The model under review builds one solid part; all positions refer to its coordinate system, in mm. Round coordinates to 2 decimals unless told otherwise and drop trailing zeros. Write each loop counter-clockwise with the first axis right and the second up, starting at its lowest first coordinate (ties: lowest second). Pieces come first, ordered by that corner, then holes. Notation, with made-up numbers: (23, 22) - (73, 22) arc R17 ccw to (73, 31) - close; hole circle Ø4 at (19, -6.5). An arc over 180 degrees is marked (long way). Use one line per item in the form item = value.
from build123d import *

# Parameters (mm, degrees)
SKETCH_1_W          = 31.5
SKETCH_1_H          = 31.5
EXTRUDE_1_DEPTH     = 0.2
SKETCH_2_R          = 4.5
CUT_EXTRUDE_1_DEPTH = 10
SKETCH_3_R          = 1.5
SKETCH_3_R_2        = 4.5
CUT_EXTRUDE_2_DEPTH = 0.2


with BuildPart() as part:
    # 스케치1 → 보스-돌출1 (new body)
    with BuildSketch(Plane.XY):
        with Locations((15.75, 15.75)):
            Rectangle(SKETCH_1_W, SKETCH_1_H)
    extrude(amount=EXTRUDE_1_DEPTH)

    # 스케치2 → 컷-돌출1 (cut)
    with BuildSketch(Plane.XY.offset(0.2)):
        with Locations((15.75, 15.75)):
            Circle(SKETCH_2_R)
    extrude(amount=-CUT_EXTRUDE_1_DEPTH, mode=Mode.SUBTRACT)

    # 스케치3 → 컷-돌출2 (cut)
    with BuildSketch(Plane.XY.offset(0.2)):
        with Locations((29.7, 15.75)):
            Circle(SKETCH_3_R)
        with Locations((15.75, 15.75)):
            Circle(SKETCH_3_R_2)
        with Locations((15.75, 1.8)):
            Circle(SKETCH_3_R)
        with Locations((1.8, 15.75)):
            Circle(SKETCH_3_R)
        with Locations((15.75, 29.7)):
            Circle(SKETCH_3_R)
        with Locations((1.8, 29.7)):
            Circle(SKETCH_3_R)
        with Locations((29.7, 29.7)):
            Circle(SKETCH_3_R)
        with Locations((29.7, 1.8)):
            Circle(SKETCH_3_R)
        with Locations((1.8, 1.8)):
            Circle(SKETCH_3_R)
    extrude(amount=-CUT_EXTRUDE_2_DEPTH, mode=Mode.SUBTRACT)


solid = part.part
(1) Add section C-C on y = 1.8. Write out the cut boundary in (x, z).
Geometry results:
outline = (0, 0) - (0.3, 0) - (0.3, 0.2) - (0, 0.2) - close; (3.3, 0) - (14.25, 0) - (14.25, 0.2) - (3.3, 0.2) - close; (17.25, 0) - (28.2, 0) - (28.2, 0.2) - (17.25, 0.2) - close; (31.2, 0) - (31.5, 0) - (31.5, 0.2) - (31.2, 0.2) - close
(2) Add section B-B on x = 15.75. Write out the cut boundary in (y, z).
Geometry results:
outline = (0, 0) - (0.3, 0) - (0.3, 0.2) - (0, 0.2) - close; (3.3, 0) - (11.25, 0) - (11.25, 0.2) - (3.3, 0.2) - close; (20.25, 0) - (28.2, 0) - (28.2, 0.2) - (20.25, 0.2) - close; (31.2, 0) - (31.5, 0) - (31.5, 0.2) - (31.2, 0.2) - close
(3) Insertion check: P1, Ø2.5, axis at x = 1.8, y = 29.7, coming from the +Z side. The pin has a flat end and moves straight along its axis. Give the tip position at first contact, or say it passes through.
Geometry results:
P1 = through
(4) Add section A-A on z = 0.15. Count the separate pieces of the cut face and the enclosed holes in it, then the cut area to 3 significant figures.
Geometry results:
separate_pieces = 1
enclosed_holes = 9
area = 872 mm2
(5) To check wall thickness, follow L1, parallel to Y at x = 15.75, z = 0.1; L2, parallel to Y at x = 29.7, z = 0.15; L3, parallel to X at y = 2, z = 0.15. State the ranges of each line that lie inside material, in increasing order.
Geometry results:
L1 = 0 to 0.3, 3.3 to 11.25, 20.25 to 28.2, 31.2 to 31.5
L2 = 0 to 0.3, 3.3 to 14.25, 17.25 to 28.2, 31.2 to 31.5
L3 = 0 to 0.31, 3.29 to 14.26, 17.24 to 28.21, 31.19 to 31.5
